from build123d import *

# Parameters (mm, degrees)
SKETCH1_W           = 190
SKETCH1_H           = 50
BOSS_EXTRUDE1_DEPTH = 3
SKETCH2_R           = 14.75
SKETCH2_R_2         = 0.185342338
SKETCH2_R_3         = 2.5
CUT_EXTRUDE1_DEPTH  = 99.28021164
LPATTERN1_COUNT     = 3
LPATTERN1_PITCH     = 63.333333333
SKETCH3_W           = 190
SKETCH3_H           = 70
BOSS_EXTRUDE2_DEPTH = 3
CUT_EXTRUDE2_DEPTH  = 3
LPATTERN2_COUNT     = 3
LPATTERN2_PITCH     = 63.333333333
CUT_EXTRUDE3_DEPTH  = 1
FILLET1_R           = 20
FILLET2_R           = 20


with BuildPart() as part:
    # Sketch1 → Boss-Extrude1 (new body)
    with BuildSketch(Plane.XY):
        Rectangle(SKETCH1_W, SKETCH1_H)
    extrude(amount=BOSS_EXTRUDE1_DEPTH)

    # Sketch2 → Cut-Extrude1 (cut, through all)
    with BuildSketch(Plane.XY.offset(3)):
        with Locations((-63.333333333, 0)):
            Circle(SKETCH2_R)
        with Locations((11.583896138, 12.510607829)):
            Circle(SKETCH2_R_2)
        with Locations((-87.083333333, 0)):
            Circle(SKETCH2_R_3)
        with Locations(Location((-39.583333333, 0, 0), (0, 0, 180))):
            Circle(SKETCH2_R_3)
    cut_extrude1 = extrude(amount=-CUT_EXTRUDE1_DEPTH, mode=Mode.SUBTRACT)

    # LPattern1: Cut-Extrude1 ×3
    with Locations(*[(i * LPATTERN1_PITCH, 0, 0) for i in range(1, LPATTERN1_COUNT)]):
        add(cut_extrude1, mode=Mode.SUBTRACT)

    # Sketch3 → Boss-Extrude2 (add)
    with BuildSketch(Plane.XY.offset(3)):
        with Locations((0, 60)):
            Rectangle(SKETCH3_W, SKETCH3_H)
    extrude(amount=-BOSS_EXTRUDE2_DEPTH)

    # Sketch3<3> → Cut-Extrude2 (cut)
    with BuildSketch(Plane.XY.offset(3)):
        with BuildLine():
            Line((73.333333333, 62.2), (53.333333333, 62.2))
            ThreePointArc((53.333333333, 62.2), (51.133333333, 60), (53.333333333, 57.8))
            Line((53.333333333, 57.8), (73.333333333, 57.8))
            ThreePointArc((73.333333333, 57.8), (75.533333333, 60), (73.333333333, 62.2))
        make_face()
    cut_extrude2 = extrude(amount=-CUT_EXTRUDE2_DEPTH, mode=Mode.SUBTRACT)

    # LPattern2: Cut-Extrude2 ×3
    with Locations(*[(-i * LPATTERN2_PITCH, 0, 0) for i in range(1, LPATTERN2_COUNT)]):
        add(cut_extrude2, mode=Mode.SUBTRACT)

    # Sketch4 → Cut-Extrude3 (cut)
    with BuildSketch(Plane.XY.offset(3)):
        with BuildLine():
            Line((80.361283663, 25.5), (-80.361283663, 25.5))
            ThreePointArc((-80.361283663, 25.5), (-80.861283663, 25), (-80.361283663, 24.5))
            Line((-80.361283663, 24.5), (80.361283663, 24.5))
            ThreePointArc((80.361283663, 24.5), (80.861283663, 25), (80.361283663, 25.5))
        make_face()
    extrude(amount=-CUT_EXTRUDE3_DEPTH, mode=Mode.SUBTRACT)

    # Fillet1
    fillet1_edges = [part.edges().sort_by_distance(p)[0] for p in [
        (95, -25, 1.5),
        (-95, -25, 1.5),
    ]]
    fillet(fillet1_edges, radius=FILLET1_R)

    # Fillet2
    fillet2_edges = [part.edges().sort_by_distance(p)[0] for p in [
        (95, 95, 1.5),
        (-95, 95, 1.5),
    ]]
    fillet(fillet2_edges, radius=FILLET2_R)


solid = part.part
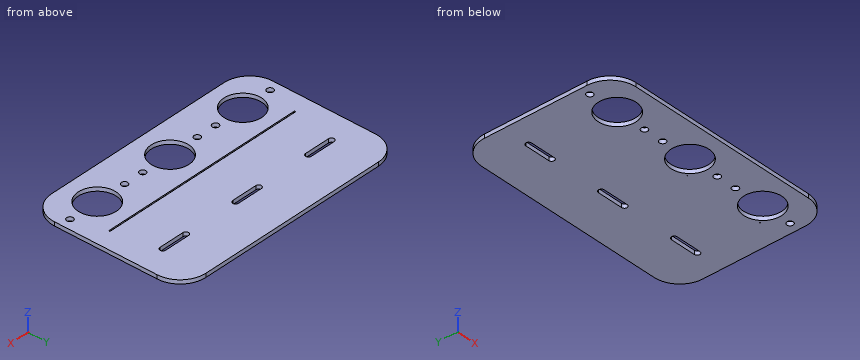
Here's how the part is built. I have some questions about the finished solid (model axes, mm). Coordinates: 2 decimals unless noted, no trailing zeros. Order: outer loops, then holes, each group sorted by start corner. A loop starts at its lowest first (then second) coordinate and runs counter-clockwise, first axis right, second up.
Item 1: If we section it at C-C on x = -23.75: List the corners of the cut face in (y, z) for me.
Result sheet:
outline: (-25, 0) - (-2.5, 0) - (-2.5, 3) - (-25, 3) - close; (2.5, 0) - (95, 0) - (95, 3) - (25.5, 3) - (25.5, 2) - (24.5, 2) - (24.5, 3) - (2.5, 3) - close
Item 2: If we section it at D-D on z = 1.5: State how many separate pieces and enclosed holes the cut face has, plus the area to 3 significant figures.
Result sheet:
separate pieces: 1
enclosed holes: 14
area: 20,000 mm2
Item 3: For P1, Ø0.8, axis at x = -8.5, y = 25, coming from the +Z side; P2, Ø23.5, axis at x = 63.33, y = 0, coming from the -Z side; P3, Ø6.5, axis at x = -39.58, y = 0, coming from the -Z side, each with a flat end and sliding along its axis, tell me the tip position at first contact or that it passes through.
Result sheet:
P1: stops at z = 2
P2: passes through
P3: stops at z = 0
Item 4: If we section it at B-B on y = 60: List the corners of the cut face in (x, z) for me, plus the area to 3 significant figures.
Result sheet:
outline: (-95, 0) - (-75.53, 0) - (-75.53, 3) - (-95, 3) - close; (-51.13, 0) - (-12.2, 0) - (-12.2, 3) - (-51.13, 3) - close; (12.2, 0) - (51.13, 0) - (51.13, 3) - (12.2, 3) - close; (75.53, 0) - (95, 0) - (95, 3) - (75.53, 3) - close
area: 350 mm2
Item 5: If we section it at A-A on x = 0: List the corners of the cut face in (y, z) for me.
Result sheet:
outline: (-25, 0) - (-14.75, 0) - (-14.75, 3) - (-25, 3) - close; (14.75, 0) - (57.8, 0) - (57.8, 3) - (25.5, 3) - (25.5, 2) - (24.5, 2) - (24.5, 3) - (14.75, 3) - close; (62.2, 0) - (95, 0) - (95, 3) - (62.2, 3) - close
Item 6: I need wall thicknesses on line 1 (Y direction, x = 0, z = 1.85); line 2 (Y direction, x = 55, z = 2.7); line 3 (Y direction, x = -9, z = 2.95). Which ranges of each line are inside material? Lowest first, please.
Result sheet:
line 1: y = -25 to -14.75, 14.75 to 57.8, 62.2 to 95
line 2: y = -25 to -12.17, 12.17 to 24.5, 25.5 to 57.8, 62.2 to 95
line 3: y = -25 to -11.69, 11.69 to 24.5, 25.5 to 57.8, 62.2 to 95
